```python
from build123d import *

# Parameters (mm, degrees)
F0_W     = 125.585321
F0_H     = 58.162786
F1_DEPTH = 25.4


with BuildPart() as f1:
    # F0 (on Front) → F1 (new body)
    with BuildSketch(Plane.XZ):
        Polygon((85.79734, 28.936708), (-51.07329, 28.936708), (-51.07329, -39.643291), (85.80731, -39.643291), align=None)
        with Locations((18.664179, -6.510761)):
            Rectangle(F0_W, F0_H, mode=Mode.SUBTRACT)
    extrude(amount=F1_DEPTH)


solid = f1.part
```
Design review of the part built by this model. Coordinates are the model's own, in mm. A direction names the side the tool comes from. Give positions to 0.01 mm unless a question says otherwise; leave off trailing zeros. Loops run counter-clockwise (first coordinate to the right, second up) from the corner with the lowest first, then second, coordinate; pieces in that order, holes last. Notation, with made-up numbers: M 60.5,40.5 L 97.5,40.5 A20 ccw 97.5,48.5 Z; hole C 51,55 d10. An arc over 180 degrees is marked long. Return JSON: item names as keys, results as strings. Group by question number.
Item 1: Tool access review of faces 1 (the flat face through (16, -13, -39.643)), 2 (the flat face through (18, -13, 22.571)): name each direction out of +Z, -Z, +X, -X, +Y, -Y from which nothing blocks a thin tool from reaching the whole face with its end or side.
Item 2: We need section B-B (y = -4.25). Give the boundary of the cut face in (x, z), and give its area (3 significant figures).
Item 3: Insertion check: pin 1 Ø2 at (y, z) = (-7, 1) entering from +X. The pin has a flat end and moves straight along its axis. Give the tip position at first contact, or say it passes through.
Item 4: We need section C-C (z = 6.5). Give the boundary of the cut face in (x, y), and give its area (3 significant figures).
Item 5: We need section A-A (x = -6). Give the boundary of the cut face in (y, z).
Item 6: Mouldability with a two-part tool opening along X and no side actions: class faces 3 (the flat face through (-51.073, -13, -5)), 4 (the flat face through (81.457, -13, -7)), 5 (the flat face through (22, -25.4, 23)) as released by +X, released by -X, zero draft, split by the parting line, or undercut.
Item 7: For probe 1 along Z at (x, y) = (64.5, -14.25); probe 2 along X at (y, z) = (-13.25, 6.5), list the stretches that pass through material, from the lowest coordinate up.
Output:
{
 "1": {"face 1": "-Z, +X, -X, +Y, -Y", "face 2": "+Y, -Y"},
 "2": {"outline": "M -51.07,-39.64 L 85.81,-39.64 L 85.8,28.94 L -51.07,28.94 Z; hole M -44.13,-35.59 L 81.46,-35.59 L 81.46,22.57 L -44.13,22.57 Z", "area": "2,080 mm^2"},
 "3": {"pin 1": "stops at x = 85.8"},
 "4": {"outline": "M -51.07,-25.4 L -44.13,-25.4 L -44.13,0 L -51.07,0 Z; M 81.46,-25.4 L 85.8,-25.4 L 85.8,0 L 81.46,0 Z", "area": "287 mm^2"},
 "5": {"outline": "M -25.4,-39.64 L 0,-39.64 L 0,-35.59 L -25.4,-35.59 Z; M -25.4,22.57 L 0,22.57 L 0,28.94 L -25.4,28.94 Z"},
 "6": {"face 3": "released by -X", "face 4": "undercut", "face 5": "zero draft"},
 "7": {"probe 1": "z = -39.64 to -35.59, 22.57 to 28.94", "probe 2": "x = -51.07 to -44.13, 81.46 to 85.8"}
}
